CAD build for the part. Positions are in the model's coordinates, mm. Face numbers are marked on the shaded views. A direction names the side the tool comes from. Coordinates: 2 decimals unless noted, no trailing zeros. Order: outer loops, then holes, each group sorted by start corner. A loop starts at its lowest first (then second) coordinate and runs counter-clockwise, first axis right, second up. Notation, with made-up numbers: M 21,45 L 49,45 A23 cw 49,75 Z; hole C -37.75,-28 d9. An arc over 180 degrees is marked long. Write item = value, one per line.
from build123d import *

# Parameters (mm, degrees)
ESBO_O1_W                                           = 138
ESBO_O1_H                                           = 80
RESSALTO_EXTRUS_O1_DEPTH                            = 10
ESBO_O2_W                                           = 60
ESBO_O2_H                                           = 80
CORTE_EXTRUS_O1_DEPTH                               = 3
ESCAREADO_PARA_PARAFUSO_ALLEN_SEXTAVADO_D           = 6.6
ESCAREADO_PARA_PARAFUSO_ALLEN_SEXTAVADO_CSINK_D     = 13.44
ESCAREADO_PARA_PARAFUSO_ALLEN_SEXTAVADO_CSINK_ANGLE = 90
CHANFRO1_SIZE                                       = 5
CHANFRO2_SIZE                                       = 3


with BuildPart() as part:
    # Esboço1 → Ressalto-extrusão1 (new body)
    with BuildSketch(Plane.XY):
        with Locations((-69, 40)):
            Rectangle(ESBO_O1_W, ESBO_O1_H)
    extrude(amount=RESSALTO_EXTRUS_O1_DEPTH)

    # Esboço2 → Corte-extrusão1 (cut)
    with BuildSketch(Plane.XY.offset(10)):
        with Locations((-30, 40)):
            Rectangle(ESBO_O2_W, ESBO_O2_H)
    extrude(amount=-CORTE_EXTRUS_O1_DEPTH, mode=Mode.SUBTRACT)

    # Escareado para parafuso Allen sextavado escareado de M62 (through all)
    with Locations(Plane(origin=(0, 0, 0), x_dir=(-1, 0, 0), z_dir=(0, 0, -1))):
        with Locations((10, 60), (42, 60), (42, 18), (10, 18)):
            CounterSinkHole(ESCAREADO_PARA_PARAFUSO_ALLEN_SEXTAVADO_D / 2, ESCAREADO_PARA_PARAFUSO_ALLEN_SEXTAVADO_CSINK_D / 2, counter_sink_angle=ESCAREADO_PARA_PARAFUSO_ALLEN_SEXTAVADO_CSINK_ANGLE)

    # Chanfro1
    chanfro1_edges = [part.edges().sort_by_distance(p)[0] for p in [
        (-30, 0, 7),
    ]]
    chamfer(chanfro1_edges, length=CHANFRO1_SIZE)

    # Chanfro2
    chanfro2_edges = [part.edges().sort_by_distance(p)[0] for p in [
        (-138, 40, 10),
        (-138, 40, 0),
    ]]
    chamfer(chanfro2_edges, length=CHANFRO2_SIZE)


solid = part.part
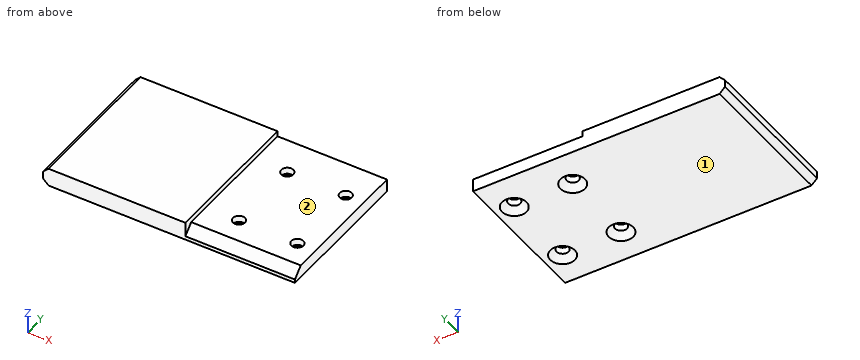
(1) Slice it at C-C, the plane y = 30. Write the cut outline in (x, z).
Evaluation:
outline = M -138,3 L -135,0 L 0,0 L 0,7 L -60,7 L -60,10 L -135,10 L -138,7 Z
(2) Slice it at B-B, the plane y = 18. Write the cut outline in (x, z), then the cut area to 3 significant figures.
Evaluation:
outline = M -138,3 L -135,0 L -48.72,0 L -45.3,3.42 L -45.3,7 L -60,7 L -60,10 L -135,10 L -138,7 Z; M -38.7,3.42 L -35.28,0 L -16.72,0 L -13.3,3.42 L -13.3,7 L -38.7,7 Z; M -6.7,3.42 L -3.28,0 L 0,0 L 0,7 L -6.7,7 Z
area = 1,080 mm²
(3) Tool access for the marked faces 1 and 2: list every direction of +Z, -Z, +X, -X, +Y, -Y with a clear straight run to the whole face (end or side of a thin tool).
Evaluation:
face_1 = -Z, +X, -X, +Y, -Y
face_2 = +Z, +X, +Y, -Y
(4) Wall check: line 1 (X direction, y = 18, z = 5.2); line 2 (Y direction, x = -42, z = 5.45); line 3 (Y direction, x = -10, z = 4.6). Give the ranges that are in metal, low to high. Write a range as from..to.
Evaluation:
line_1 = -138..-45.3, -38.7..-13.3, -6.7..0
line_2 = 3.45..14.7, 21.3..56.7, 63.3..80
line_3 = 2.6..14.7, 21.3..56.7, 63.3..80
(5) Slice it at D-D, the plane x = -27.5. Write the cut outline in (y, z).
Evaluation:
outline = M 0,0 L 80,0 L 80,7 L 5,7 L 0,2 Z
(6) Pin check, flat tips, straight feed: pin 1 Ø7.5 at (x, y) = (-42, 60) entering from +Z; pin 2 Ø4 at (x, y) = (-10, 60) entering from -Z; pin 3 Ø10.5 at (x, y) = (-10, 18) entering from -Z; pin 4 Ø5 at (x, z) = (-57, 8) entering from -Y. Stop position of each tip, or through.
Evaluation:
pin_1 = 7
pin_2 = through
pin_3 = 1.47
pin_4 = 3.5
(7) Slice it at A-A, the plane x = -42. Write the cut outline in (y, z), then the cut area to 3 significant figures.
Evaluation:
outline = M 0,0 L 11.28,0 L 14.7,3.42 L 14.7,7 L 5,7 L 0,2 Z; M 21.3,3.42 L 24.72,0 L 53.28,0 L 56.7,3.42 L 56.7,7 L 21.3,7 Z; M 63.3,3.42 L 66.72,0 L 80,0 L 80,7 L 63.3,7 Z
area = 432 mm²
